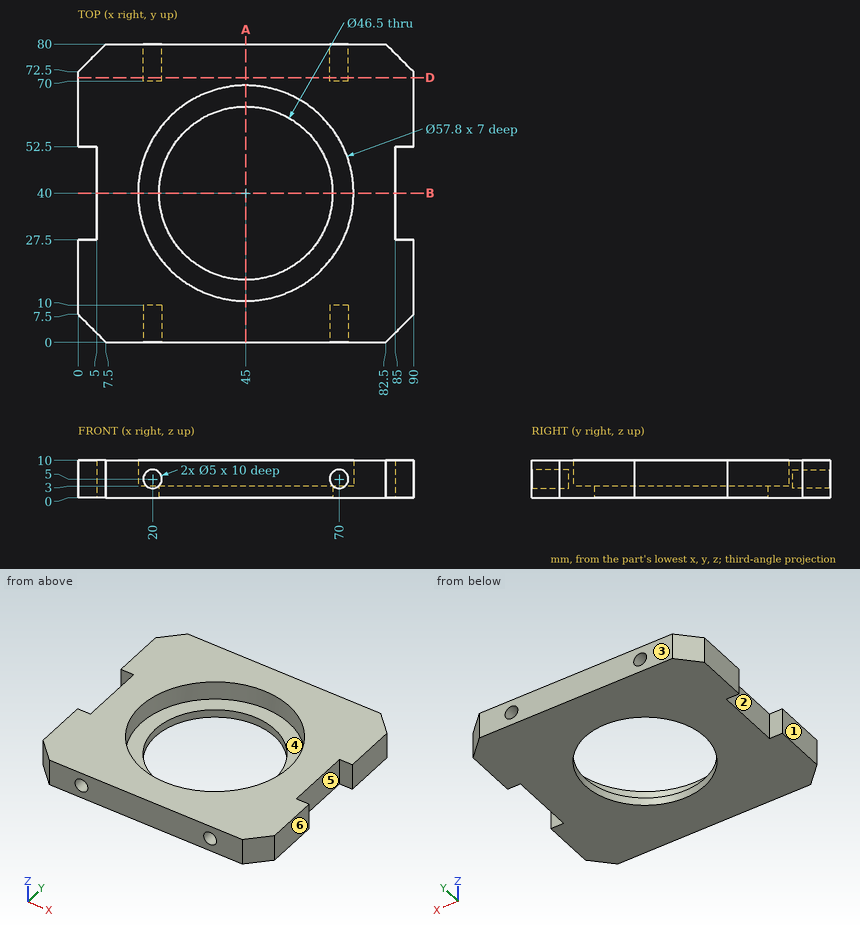
Drawing for the job (mm, zero at the part's lowest x, y, z). A direction names the side the tool comes from. Give positions to 0.01 mm unless a question says otherwise; leave off trailing zeros. Order: outer loops, then holes, each group sorted by start corner. A loop starts at its lowest first (then second) coordinate and runs counter-clockwise, first axis right, second up. Notation, with made-up numbers: M 68.5,59 L 119.5,59 A28 cw 119.5,84 Z; hole C 22.5,-7 d9. An arc over 180 degrees is marked long. Use a Markdown table: item, result. Add a question column.
(1) 3-axis set-ups, long thin cutter, end or side, ignore diameter. For the marked faces 4, 5 and 6: which of +Z, -Z, +X, -X, +Y, -Y reach the whole face in a straight line?
(2) Saw through at A-A, the plane x = 45. Give the cut face in (y, z), and give its area (3 significant figures).
(3) Drop flat-ended pins along their axis: P1, Ø5.5, axis at x = 87.5, z = 5, coming from the +Y side; P2, Ø5, axis at y = 39.5, z = 3, coming from the -X side; P3, Ø1.5, axis at x = 19.5, z = 6, coming from the +Y side. Give the stop position or say it passes through.
(4) Mould opens along Y. For the marked faces 1, 2 and 3 say: +Y half, -Y half, draft (parallel to the pull), parting line (faces both ways), or undercut.
(5) Saw through at B-B, the plane y = 40. Give the cut face in (x, z), and give its area (3 significant figures).
(6) Saw through at D-D, the plane y = 71. Give the cut face in (x, z), and give its area (3 significant figures).
(7) Probe line 1 along Z through (x, y) = (70, 72); line 2 along X through (y, z) = (6, 6); line 3 along X through (y, z) = (5, 3.25). List the from-to ranges inside material, lowest first. Write a range as [from, to].
Answer key:
| question | item | result |
|---|---|---|
| 1 | face 4 | +Z |
| 1 | face 5 | +Z, -Z, +X |
| 1 | face 6 | +Z, -Z, +X, +Y, -Y |
| 2 | outline | M 0,0 L 16.75,0 L 16.75,3 L 11.1,3 L 11.1,10 L 0,10 Z; M 63.25,0 L 80,0 L 80,10 L 68.9,10 L 68.9,3 L 63.25,3 Z |
| 2 | area | 256 mm^2 |
| 3 | P1 | y = 77.75 |
| 3 | P2 | x = 5 |
| 3 | P3 | y = 70 |
| 4 | face 1 | draft |
| 4 | face 2 | undercut |
| 4 | face 3 | +Y half |
| 5 | outline | M 5,0 L 21.75,0 L 21.75,3 L 16.1,3 L 16.1,10 L 5,10 Z; M 68.25,0 L 85,0 L 85,10 L 73.9,10 L 73.9,3 L 68.25,3 Z |
| 5 | area | 256 mm^2 |
| 6 | outline | M 0,0 L 90,0 L 90,10 L 0,10 Z; hole C 20,5 d5; hole C 70,5 d5 |
| 6 | area | 861 mm^2 |
| 7 | line 1 | [0, 2.5], [7.5, 10] |
| 7 | line 2 | [1.5, 17.71], [22.29, 67.71], [72.29, 88.5] |
| 7 | line 3 | [2.5, 18.21], [21.79, 68.21], [71.79, 87.5] |
